Input: part model. Units: mm. Frame: model coordinates. Face numbers are marked on the shaded views. A direction names the side the tool comes from. Give positions to 0.01 mm unless a question says otherwise; leave off trailing zeros. Loops run counter-clockwise (first coordinate to the right, second up) from the corner with the lowest first, then second, coordinate; pieces in that order, holes last. Notation, with made-up numbers: M 39,15.25 L 72,15.25 A18 ccw 72,23.25 Z; hole C 79,37.5 d6. An arc over 180 degrees is marked long. One line per item, written item: value. Start each with the question number.
(1) Pin query (flat end, axial travel): P1, Ø4, axis at x = -25.5, y = -4, coming from the -Z side; P2, Ø6, axis at y = -8.5, z = 6, coming from the -X side; P3, Ø0.7, axis at x = -11.5, z = 24.5, coming from the +Y side. Return the tip coordinate at first contact, or that it passes through.
(2) Section C-C on x = -14. Output: boundary loops of the cut face in (y, z), plus the area to 3 significant figures.
(3) Pull-direction query (Z, two-part tool) for the marked faces 1, 2, 3 and 4; classes: released by +Z, released by -Z, zero draft, split by the parting line, or undercut.
(4) Section B-B on y = -1.75. Output: boundary loops of the cut face in (x, z), plus the area to 3 significant figures.
(5) Ray query, line 1 along Z through (x, y) = (-8, -9.25); line 2 along Z through (x, y) = (-17.5, -2.25); line 3 along X through (y, z) = (-10.75, 5.5). Return the intervals inside material, ascending. Write a range as from..to.
(6) Section D-D on z = 12.5. Output: boundary loops of the cut face in (x, y), plus the area to 3 significant figures.
(7) Access query for the marked faces 5, 6, 7 and 8. Directions: +Z, -Z, +X, -X, +Y, -Y. A direction counts if a zero-diameter tool reaches every point of the face in a straight line with its end or side. Return the directions, or none.
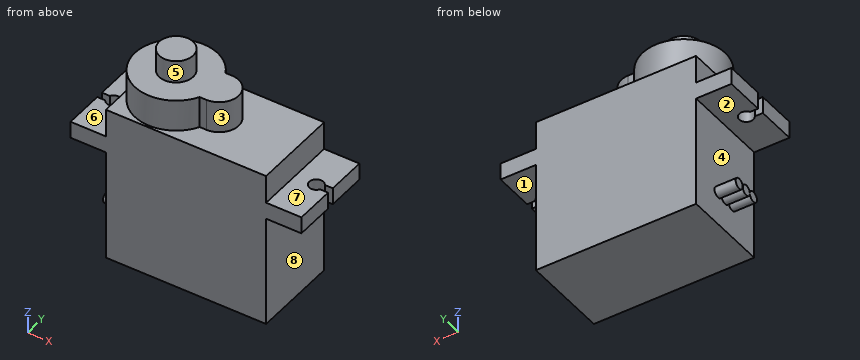
```python
from build123d import *

# Parameters (mm, degrees)
SZKIC1_W                         = 22.7
SZKIC1_H                         = 12.3
DODANIE_WYCI_GNI_CIE1_DEPTH      = 22.2
DODANIE_WYCI_GNI_CIE2_DEPTH      = 5
DODANIE_WYCI_GNI_CIE2_DEPTH_BACK = 27.7
SZKIC2_W                         = 2.4
SZKIC2_H                         = 12.3
DODANIE_WYCI_GNI_CIE3_DEPTH      = 4.5
SZKIC8_R                         = 2.4
DODANIE_WYCI_GNI_CIE4_DEPTH      = 3.2
WYTNIJ_WYCI_GNI_CIE1_DEPTH       = 2.4
WYTNIJ_WYCI_GNI_CIE2_DEPTH       = 2.4
SZKIC11_R                        = 0.75
DODANIE_WYCI_GNI_CIE8_DEPTH      = 25.7


with BuildPart() as part:
    # Szkic1 → Dodanie-wyciągnięcie1 (new body)
    with BuildSketch(Plane.XY):
        with Locations((-11.570890411, -6.425490196)):
            Rectangle(SZKIC1_W, SZKIC1_H)
    extrude(amount=DODANIE_WYCI_GNI_CIE1_DEPTH)

    # Szkic2 → Dodanie-wyciągnięcie2 (add, two sides: drawn at the far end of the back side and taken through both)
    with BuildSketch(Plane(origin=(-0.220890411, 0, 0), x_dir=(0, 0, -1), z_dir=(1, 0, 0)).offset(-DODANIE_WYCI_GNI_CIE2_DEPTH_BACK)):
        with Locations((-17, -6.425490196)):
            Rectangle(SZKIC2_W, SZKIC2_H)
    extrude(amount=DODANIE_WYCI_GNI_CIE2_DEPTH + DODANIE_WYCI_GNI_CIE2_DEPTH_BACK)

    # Szkic3 → Dodanie-wyciągnięcie3 (add)
    with BuildSketch(Plane.XY.offset(22.2)):
        with BuildLine():
            Line((-10.970890411, -9.175490196), (-11.907558154, -9.175490196))
            ThreePointArc((-11.907558154, -9.175490196), (-22.920890411, -6.425490196), (-11.907558154, -3.675490196))
            Line((-11.907558154, -3.675490196), (-10.970890411, -3.675490196))
            ThreePointArc((-10.970890411, -3.675490196), (-8.220890411, -6.425490196), (-10.970890411, -9.175490196))
        make_face()
    extrude(amount=DODANIE_WYCI_GNI_CIE3_DEPTH)

    # Szkic8 → Dodanie-wyciągnięcie4 (add)
    with BuildSketch(Plane.XY.offset(26.7)):
        with Locations((-17.070890411, -6.425490196)):
            Circle(SZKIC8_R)
    extrude(amount=DODANIE_WYCI_GNI_CIE4_DEPTH)

    # Szkic9 → Wytnij-wyciągnięcie1 (cut)
    with BuildSketch(Plane.XY.offset(18.2)):
        with BuildLine():
            Line((4.779109589, -6.425490196), (4.779109589, -5.925490196))
            Line((4.779109589, -5.925490196), (3.645134993, -5.925490196))
            ThreePointArc((3.645134993, -5.925490196), (1.779109589, -6.425490196), (3.645134993, -6.925490196))
            Line((3.645134993, -6.925490196), (4.779109589, -6.925490196))
            Line((4.779109589, -6.925490196), (4.779109589, -6.425490196))
        make_face()
    extrude(amount=-WYTNIJ_WYCI_GNI_CIE1_DEPTH, mode=Mode.SUBTRACT)

    # Szkic10 → Wytnij-wyciągnięcie2 (cut)
    with BuildSketch(Plane.XY.offset(18.2)):
        with BuildLine():
            Line((-27.920890411, -5.925490196), (-27.920890411, -6.925490196))
            Line((-27.920890411, -6.925490196), (-26.786915815, -6.925490196))
            ThreePointArc((-26.786915815, -6.925490196), (-24.920890411, -6.425490196), (-26.786915815, -5.925490196))
            Line((-26.786915815, -5.925490196), (-27.920890411, -5.925490196))
        make_face()
    extrude(amount=-WYTNIJ_WYCI_GNI_CIE2_DEPTH, mode=Mode.SUBTRACT)

    # Szkic11 → Dodanie-wyciągnięcie8 (add)
    with BuildSketch(Plane(origin=(-0.220890411, 0, 0), x_dir=(0, 0, -1), z_dir=(1, 0, 0))):
        with Locations((-4.75, -6.425490196)):
            Circle(SZKIC11_R)
        with Locations((-4.75, -4.915490196)):
            Circle(SZKIC11_R)
        with Locations((-4.75, -7.935490196)):
            Circle(SZKIC11_R)
    extrude(amount=-DODANIE_WYCI_GNI_CIE8_DEPTH)


solid = part.part
```
Output values:
1. P1: stops at z = 4
1. P2: stops at x = -25.92
1. P3: stops at y = -3.68
2. outline: M -12.58,0 L -0.28,0 L -0.28,22.2 L -1.45,22.2 L -1.45,26.7 L -11.4,26.7 L -11.4,22.2 L -12.58,22.2 Z
2. area: 318 mm²
3. face 1: released by -Z
3. face 2: undercut
3. face 3: zero draft
3. face 4: undercut
4. outline: M -27.92,15.8 L -22.92,15.8 L -22.92,0 L -0.22,0 L -0.22,15.8 L 4.78,15.8 L 4.78,18.2 L -0.22,18.2 L -0.22,22.2 L -13.55,22.2 L -13.55,26.7 L -20.59,26.7 L -20.59,22.2 L -22.92,22.2 L -22.92,18.2 L -27.92,18.2 Z
4. area: 560 mm²
5. line 1: z = 0..22.2
5. line 2: z = 0..26.7
5. line 3: x = -22.92..-0.22
6. outline: M -22.92,-12.58 L -0.22,-12.58 L -0.22,-0.28 L -22.92,-0.28 Z
6. area: 279 mm²
7. face 5: +Z
7. face 6: +Z, -X, +Y, -Y
7. face 7: +Z, +X, +Y, -Y
7. face 8: -Z, +X, +Y, -Y
